```python
from build123d import *

# Parameters (mm, degrees)
F1_DEPTH = 40
F2_W     = 20
F2_H     = 3
F3_DEPTH = 25


with BuildPart() as f1:
    # F0 (on Top) → F1 (new body)
    with BuildSketch(Plane.XY):
        with BuildLine():
            ThreePointArc((0, 4), (1.171573, 1.171573), (4, 0))
            Line((4, 0), (126, 0))
            ThreePointArc((126, 0), (128.828427, 1.171573), (130, 4))
            Line((130, 4), (130, 49))
            ThreePointArc((130, 49), (128.828427, 51.828427), (126, 53))
            Line((126, 53), (4, 53))
            ThreePointArc((4, 53), (1.171573, 51.828427), (0, 49))
            Line((0, 49), (0, 4))
        make_face()
    extrude(amount=F1_DEPTH)

    # F2 (on face) → F3 (cut)
    with BuildSketch(Plane.XY.offset(40)):
        with Locations((15, 46.5)):
            Rectangle(F2_W, F2_H)
        with Locations((15.066508, 38.500276)):
            Rectangle(F2_W, F2_H)
        with Locations((15.133017, 30.500553)):
            Rectangle(F2_W, F2_H)
        with Locations((15.199525, 22.500829)):
            Rectangle(F2_W, F2_H)
        with Locations((15.266034, 14.501106)):
            Rectangle(F2_W, F2_H)
        with Locations((15.332542, 6.501382)):
            Rectangle(F2_W, F2_H)
        with Locations((40, 46.5)):
            Rectangle(F2_W, F2_H)
        with Locations((40.066508, 38.500276)):
            Rectangle(F2_W, F2_H)
        with Locations((40.133017, 30.500553)):
            Rectangle(F2_W, F2_H)
        with Locations((40.199525, 22.500829)):
            Rectangle(F2_W, F2_H)
        with Locations((40.266034, 14.501106)):
            Rectangle(F2_W, F2_H)
        with Locations((40.332542, 6.501382)):
            Rectangle(F2_W, F2_H)
        with Locations((65, 46.5)):
            Rectangle(F2_W, F2_H)
        with Locations((65.066508, 38.500276)):
            Rectangle(F2_W, F2_H)
        with Locations((65.133017, 30.500553)):
            Rectangle(F2_W, F2_H)
        with Locations((65.199525, 22.500829)):
            Rectangle(F2_W, F2_H)
        with Locations((65.266034, 14.501106)):
            Rectangle(F2_W, F2_H)
        with Locations((65.332542, 6.501382)):
            Rectangle(F2_W, F2_H)
        with Locations((90, 46.5)):
            Rectangle(F2_W, F2_H)
        with Locations((90.066508, 38.500276)):
            Rectangle(F2_W, F2_H)
        with Locations((90.133017, 30.500553)):
            Rectangle(F2_W, F2_H)
        with Locations((90.199525, 22.500829)):
            Rectangle(F2_W, F2_H)
        with Locations((90.266034, 14.501106)):
            Rectangle(F2_W, F2_H)
        with Locations((90.332542, 6.501382)):
            Rectangle(F2_W, F2_H)
        with Locations((115, 46.5)):
            Rectangle(F2_W, F2_H)
        with Locations((115.066508, 38.500276)):
            Rectangle(F2_W, F2_H)
        with Locations((115.133017, 30.500553)):
            Rectangle(F2_W, F2_H)
        with Locations((115.199525, 22.500829)):
            Rectangle(F2_W, F2_H)
        with Locations((115.266034, 14.501106)):
            Rectangle(F2_W, F2_H)
        with Locations((115.332542, 6.501382)):
            Rectangle(F2_W, F2_H)
    extrude(amount=-F3_DEPTH, mode=Mode.SUBTRACT)


solid = f1.part
```
For this review, take the finished solid that the model builds, in its own axes (mm). Round coordinates to 2 decimals unless told otherwise and drop trailing zeros. Write each loop counter-clockwise with the first axis right and the second up, starting at its lowest first coordinate (ties: lowest second). Pieces come first, ordered by that corner, then holes.
1) Take a section at B-B on x = 122. Give the boundary of the cut face in (y, z), then the cut area to 3 significant figures.
Answer below:
outline: (0, 0) - (53, 0) - (53, 40) - (48, 40) - (48, 15) - (45, 15) - (45, 40) - (40, 40) - (40, 15) - (37, 15) - (37, 40) - (32, 40) - (32, 15) - (29, 15) - (29, 40) - (24, 40) - (24, 15) - (21, 15) - (21, 40) - (16, 40) - (16, 15) - (13, 15) - (13, 40) - (8, 40) - (8, 15) - (5, 15) - (5, 40) - (0, 40) - close
area: 1,670 mm2
2) Take a section at A-A on z = 18. State how many separate pieces and enclosed holes the cut face has, then the cut area to 3 significant figures.
Answer below:
separate pieces: 1
enclosed holes: 30
area: 5,080 mm2
3) For line 1 along X through (y, z) = (30.5, 22); line 2 along X through (y, z) = (7, 18); line 3 along Z through (x, y) = (9, 46), list the stretches that pass through material, from the lowest coordinate up.
Answer below:
line 1: x = 0 to 5.13, 25.13 to 30.13, 50.13 to 55.13, 75.13 to 80.13, 100.13 to 105.13, 125.13 to 130
line 2: x = 0 to 5.33, 25.33 to 30.33, 50.33 to 55.33, 75.33 to 80.33, 100.33 to 105.33, 125.33 to 130
line 3: z = 0 to 15
4) Mouldability with a two-part tool opening along X and no side actions: class faces 1 (the face through (90, 31, 15)), 2 (the face through (66, 53, 20)) as +X half, -X half, draft (parallel to the pull), parting line (faces both ways), or undercut.
Answer below:
face 1: undercut
face 2: draft
5) Insertion check: pin 1 Ø0.9 at (x, y) = (113, 31) entering from +Z. The pin has a flat end and moves straight along its axis. Give the tip position at first contact, or say it passes through.
Answer below:
pin 1: stops at z = 15
